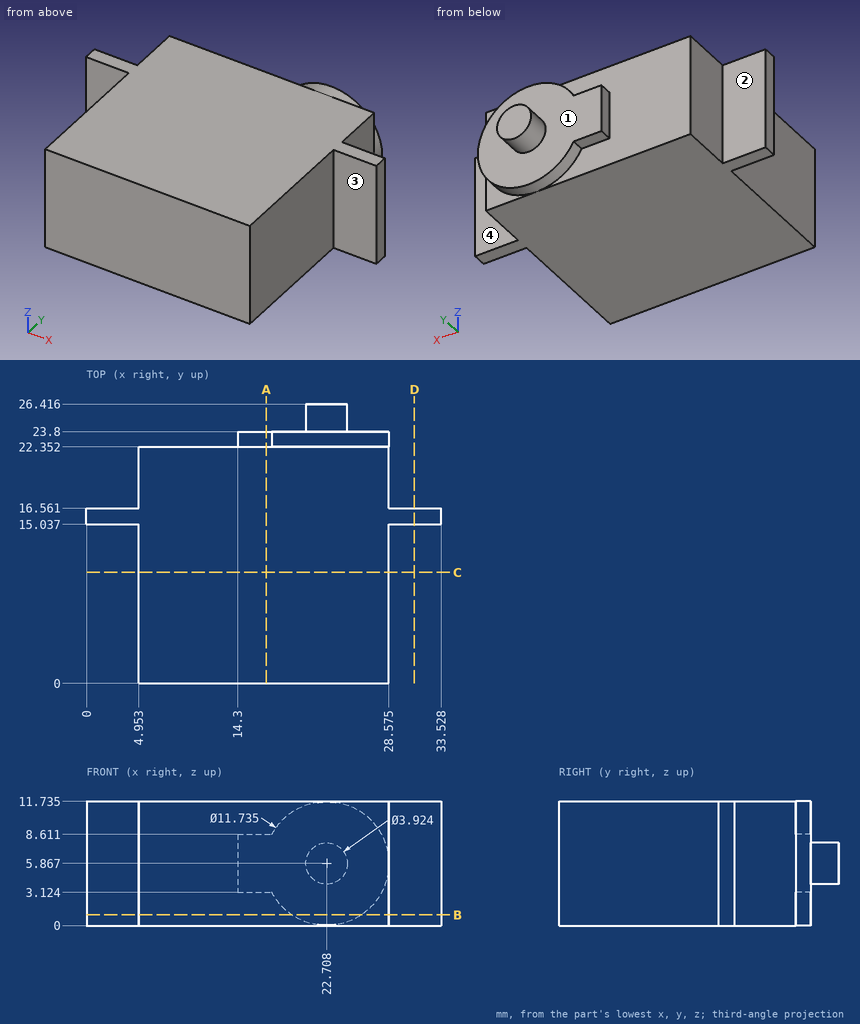
Part print with two shaded views. Sizes in mm from the minimum x, y, z corner. A direction names the side the tool comes from. Coordinates: 2 decimals unless noted, no trailing zeros. Order: outer loops, then holes, each group sorted by start corner. A loop starts at its lowest first (then second) coordinate and runs counter-clockwise, first axis right, second up.
(1) Saw through at C-C, the plane y = 10.5. Write the cut outline in (x, z) (1 decimal).
Solution:
outline: (5, 0) - (28.6, 0) - (28.6, 11.7) - (5, 11.7) - close
(2) Saw through at B-B, the plane z = 1. Write the cut outline in (x, y) (1 decimal).
Solution:
outline: (0, 15) - (5, 15) - (5, 0) - (28.6, 0) - (28.6, 15) - (33.5, 15) - (33.5, 16.6) - (28.6, 16.6) - (28.6, 22.4) - (26, 22.4) - (26, 23.8) - (19.4, 23.8) - (19.4, 22.4) - (5, 22.4) - (5, 16.6) - (0, 16.6) - close
(3) Saw through at A-A, the plane x = 17. Write the cut outline in (y, z) (1 decimal), and give its area (3 significant figures).
Solution:
outline: (0, 0) - (22.4, 0) - (22.4, 3.1) - (23.8, 3.1) - (23.8, 8.6) - (22.4, 8.6) - (22.4, 11.7) - (0, 11.7) - close
area: 270 mm2
(4) Saw through at D-D, the plane x = 31. Write the cut outline in (y, z) (1 decimal), and give its area (3 significant figures).
Solution:
outline: (15, 0) - (16.6, 0) - (16.6, 11.7) - (15, 11.7) - close
area: 17.9 mm2
(5) Drill centre lines: L1, parallel to X at y = 22, z = 11.25 (1 decimal); L2, parallel to Y at x = 11, z = 3.5; L3, parallel to Y at x = 20, z = 6. Where is each one in solid material? Low to high.
Solution:
L1: x = 5 to 28.6
L2: y = 0 to 22.35
L3: y = 0 to 23.8
(6) Which spindle directions (+Z, -Z, +X, -X, +Y, -Y) get a long thin tool onto all of the face, cutting with end or side? Do the marked faces 1, 2, 3 and 4. Say none if no direction does.
Solution:
face 1: +Y
face 2: +Z, -Z, -X, +Y
face 3: +Z, -Z, +X, -Y
face 4: +Z, -Z, +X, +Y
(7) Pin check, flat tips, straight feed: pin 1 Ø2 at (y, z) = (8, 10.5) entering from +X (3 decimals); pin 2 Ø2.5 at (x, z) = (32, 6) entering from -Y; pin 3 Ø1.8 at (x, z) = (27, 8.5) entering from +Y. Stop position of each tip, or through.
Solution:
pin 1: stops at x = 28.575
pin 2: stops at y = 15.04
pin 3: stops at y = 23.8
